```python
from build123d import *

# Parameters (mm, degrees)
BASE_W                = 72.33
BASE_H                = 80
MAIN_DEPTH            = 3
GEAR_AXIS_HOLES_D     = 5.7
CHAMFER1_SIZE         = 3.5
FILLET6_R             = 3
F_2_CLEARANCE_HOLE2_D = 2.4384
BOSS_EXTRUDE4_DEPTH   = 3


with BuildPart() as part:
    # Base → Main (new body)
    with BuildSketch(Plane.XY):
        with Locations((7.059154817, 0)):
            Rectangle(BASE_W, BASE_H)
    extrude(amount=MAIN_DEPTH)

    # Gear Axis Holes (through all)
    with Locations(Plane(origin=(0, 0, 3), x_dir=(-1, 0, 0), z_dir=(0, 0, 1))):
        with Locations((22.605845183, 20), (22.605845183, -20)):
            Hole(GEAR_AXIS_HOLES_D / 2)

    # Chamfer1
    chamfer1_edges = [part.edges().sort_by_distance(p)[0] for p in [
        (-29.105845183, -40, 1.5),
        (-29.105845183, 40, 1.5),
    ]]
    chamfer(chamfer1_edges, length=CHAMFER1_SIZE)

    # Fillet6
    fillet6_edges = [part.edges().sort_by_distance(p)[0] for p in [
        (-25.605845183, -40, 1.5),
        (-29.105845183, 36.5, 1.5),
        (-29.105845183, -36.5, 1.5),
        (-25.605845183, 40, 1.5),
        (43.224154817, 40, 1.5),
        (43.224154817, -40, 1.5),
    ]]
    fillet(fillet6_edges, radius=FILLET6_R)

    # #2 Clearance Hole2 (through all)
    with Locations(Plane.XY.offset(3)):
        with Locations((9.099154817, 35), (38.224154817, 35), (38.224154817, -35)):
            Hole(F_2_CLEARANCE_HOLE2_D / 2)

    # Sketch24 → Boss-Extrude4 (add)
    with BuildSketch(Plane.XY.offset(3)):
        with BuildLine():
            Line((-29.105845183, 28.874119675), (-29.105845183, 11.125880325))
            ThreePointArc((-29.105845183, 11.125880325), (-33.605845183, 20), (-29.105845183, 28.874119675))
        make_face()
        with BuildLine():
            Line((-29.105845183, -11.125880325), (-29.105845183, -28.874119675))
            ThreePointArc((-29.105845183, -28.874119675), (-33.605845183, -20), (-29.105845183, -11.125880325))
        make_face()
    extrude(amount=-BOSS_EXTRUDE4_DEPTH)


solid = part.part
```
Geometry check sheet. Reference: the model listing, model coordinates, mm. A direction names the side the tool comes from. Coordinates: 2 decimals unless noted, no trailing zeros. Order: outer loops, then holes, each group sorted by start corner. A loop starts at its lowest first (then second) coordinate and runs counter-clockwise, first axis right, second up.
Item 1: Mould release check, pull along X, two halves, no side actions. Record for faces 1 (the flat face through (7, -40, 1)), 2 (the cylindrical face through (-33.605, -20.145, 1.521)), 3 (the cylindrical face through (42.322, -39.145, 1.521)), 4 (the cylindrical face through (37.1, -35.47, 1.48)): released by +X, released by -X, zero draft, split by the parting line, or undercut.
Item 2: Section check B-B (z = 1.1). Enter the section's corners in (x, y).
Item 3: Section check C-C (y = -30). Enter the section's corners in (x, z), plus the area to 3 significant figures.
Item 4: Depth check by flat-ended pin: pin 1 (1.5 mm diameter, centred on y = 23.5, z = 2, fed in from -X). Enter the tip coordinate at first touch or a pass-through.
Item 5: Scan lines: line 1 along X through (y, z) = (-20, 1.95); line 2 along X through (y, z) = (-2, 0.2); line 3 along X through (y, z) = (21, 1.9). Record each from-to range of solid material in increasing order.
Item 6: Section check A-A (y = 20). Enter the section's corners in (x, z).
Item 7: Tool access check on faces 5 (the flat face through (-29.106, 32, 1)), 6 (the flat face through (7, 40, 1)), 7 (the flat face through (-29.106, 0, 1)). Record the directions out of +Z, -Z, +X, -X, +Y, -Y that give a thin tool (end or side, any length) a straight path to the whole face; none if there is none.
Check sheet entries:
1. face 1: zero draft
1. face 2: released by -X
1. face 3: released by +X
1. face 4: undercut
2. outline: (-29.11, -35.26) arc R3 ccw to (-28.23, -37.38) - (-26.48, -39.12) arc R3 ccw to (-24.36, -40) - (40.22, -40) arc R3 ccw to (43.22, -37) - (43.22, 37) arc R3 ccw to (40.22, 40) - (-24.36, 40) arc R3 ccw to (-26.48, 39.12) - (-28.23, 37.38) arc R3 ccw to (-29.11, 35.26) - (-29.11, 28.87) arc R11 ccw to (-29.11, 11.13) - (-29.11, -11.13) arc R11 ccw to (-29.11, -28.87) - close; hole circle Ø5.7 at (-22.61, -20); hole circle Ø5.7 at (-22.61, 20); hole circle Ø2.44 at (9.1, 35); hole circle Ø2.44 at (38.22, -35); hole circle Ø2.44 at (38.22, 35)
3. outline: (-29.11, 0) - (43.22, 0) - (43.22, 3) - (-29.11, 3) - close
3. area: 217 mm2
4. pin 1: stops at x = -33.26
5. line 1: x = -33.61 to -25.46, -19.76 to 43.22
5. line 2: x = -29.11 to 43.22
5. line 3: x = -33.56 to -25.27, -19.94 to 43.22
6. outline: (-33.61, 0) - (-25.46, 0) - (-25.46, 3) - (-33.61, 3) - close; (-19.76, 0) - (43.22, 0) - (43.22, 3) - (-19.76, 3) - close
7. face 5: +Z, -Z, -X, +Y
7. face 6: +Z, -Z, +X, -X, +Y
7. face 7: +Z, -Z, -X
